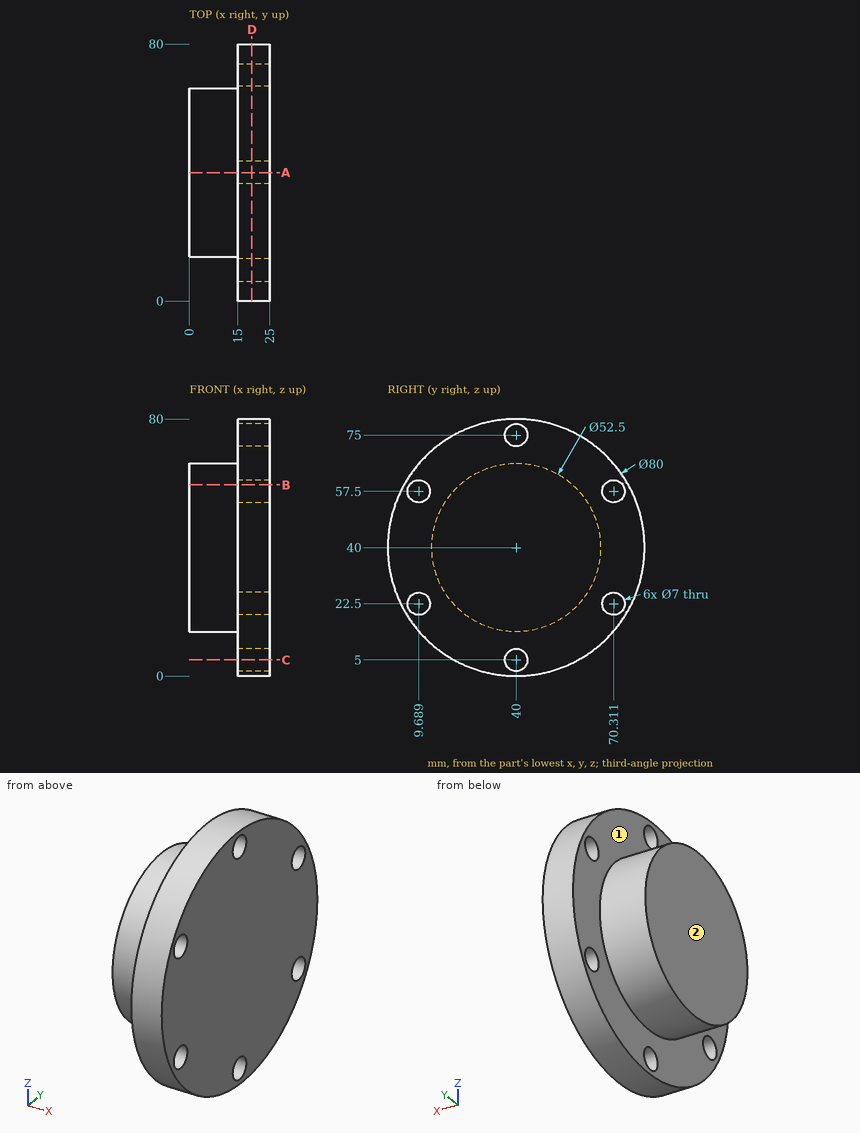
Design review of the part shown in the three views and the two pictorial views. Dimensions are in mm from the part's minimum x, y and z. A direction names the side the tool comes from. Round coordinates to 2 decimals unless told otherwise and drop trailing zeros. Order: outer loops, then holes, each group sorted by start corner. A loop starts at its lowest first (then second) coordinate and runs counter-clockwise, first axis right, second up. Notation, with made-up numbers: (30, 68.5) - (37, 68.5) arc R19 ccw to (37, 88.5) - close; hole circle Ø11 at (44, 38). An arc over 180 degrees is marked (long way). Answer in a Markdown table with one row per item.
(1) Take a section at D-D on x = 19.5. Write out the cut boundary in (y, z), plus the area to 3 significant figures.
Result set:
| item | result |
|---|---|
| outline | circle Ø80 at (40, 40); hole circle Ø7 at (9.69, 22.5); hole circle Ø7 at (9.69, 57.5); hole circle Ø7 at (40, 5); hole circle Ø7 at (40, 75); hole circle Ø7 at (70.31, 22.5); hole circle Ø7 at (70.31, 57.5) |
| area | 4,800 mm2 |
(2) Clearance check with flat-ended pins moving along their axes: P1, Ø9, axis at y = 9.69, z = 57.5, coming from the -X side; P2, Ø2, axis at x = 10.5, z = 50.5, coming from the -Y side; P3, Ø1, axis at x = 17.5, z = 71.5, coming from the -Y side; P4, Ø5.5, axis at y = 70.31, z = 22.5, coming from the +X side. State where each tip first meets the part, or that it passes through.
Result set:
| item | result |
|---|---|
| P1 | stops at x = 15 |
| P2 | stops at y = 15.53 |
| P3 | stops at y = 14.72 |
| P4 | passes through |
(3) Take a section at B-B on z = 59.5. Write out the cut boundary in (x, y) (1 decimal).
Result set:
| item | result |
|---|---|
| outline | (0, 22.4) - (15, 22.4) - (15, 12.6) - (25, 12.6) - (25, 67.4) - (15, 67.4) - (15, 57.6) - (0, 57.6) - close; (15, 5.1) - (25, 5.1) - (25, 6.8) - (15, 6.8) - close; (15, 73.2) - (25, 73.2) - (25, 74.9) - (15, 74.9) - close |
(4) Take a section at A-A on y = 40. Write out the cut boundary in (x, z), plus the area to 3 significant figures.
Result set:
| item | result |
|---|---|
| outline | (0, 13.75) - (15, 13.75) - (15, 8.5) - (25, 8.5) - (25, 71.5) - (15, 71.5) - (15, 66.25) - (0, 66.25) - close; (15, 0) - (25, 0) - (25, 1.5) - (15, 1.5) - close; (15, 78.5) - (25, 78.5) - (25, 80) - (15, 80) - close |
| area | 1,450 mm2 |
(5) Take a section at C-C on z = 5. Write out the cut boundary in (x, y) (3 decimals).
Result set:
| item | result |
|---|---|
| outline | (15, 20.635) - (25, 20.635) - (25, 36.5) - (15, 36.5) - close; (15, 43.5) - (25, 43.5) - (25, 59.365) - (15, 59.365) - close |
(6) Machinability: for the marked faces 1 and 2, which of the approach directions +Z, -Z, +X, -X, +Y, -Y give a long, thin tool a straight path to every point of the face, cutting with its end or side? Answer none if there is none.
Result set:
| item | result |
|---|---|
| face 1 | -X |
| face 2 | +Z, -Z, -X, +Y, -Y |
(7) For line 1 (Z direction, x = 22.75, y = 40); line 2 (Y direction, x = 18, z = 22.5); line 3 (Y direction, x = 24.25, z = 7) (1 decimal), list the stretches that pass through material, from the lowest coordinate up. Write a range as from..to.
Result set:
| item | result |
|---|---|
| line 1 | z = 0..1.5, 8.5..71.5, 78.5..80 |
| line 2 | y = 4.03..6.19, 13.19..66.81, 73.81..75.97 |
| line 3 | y = 17.4..37.1, 42.9..62.6 |
